Autodesk Inventor part; units mm, degrees
ref_plane "YZ Plane" through (0, 0, 0) normal (1, 0, 0) x (0, 1, 0)
ref_plane "XZ Plane" through (0, 0, 0) normal (0, 1, 0) x (-1, 0, 0)
ref_plane "XY Plane" through (0, 0, 0) normal (0, 0, 1) x (1, 0, 0)
sketch "Эскиз1" plane through (0, 0, 0) normal (0, 0, 1) x (1, 0, 0)
  circle A0 centre (0, 0) radius 3
  circle A1 centre (0, 0) radius 5
  dimension "d0" = 6
  dimension "d1" = 10
extrude "Выдавливание1" add sketch "Эскиз1" along normal blind 45
sketch "Эскиз2" plane through (0, 0, 0) normal (0, 0, -1) x (-1, 0, 0)
  circle A0 centre (0, 0) radius 13
  circle A1 centre (0, 0) radius 5
  circle A2 centre (0, 0) radius 3
  dimension "d4" = 26
extrude "Выдавливание2" add sketch "Эскиз2" along normal blind 3 contours A0 | A1
sketch "Эскиз3" plane through (0, 0, -3) normal (0, 0, -1) x (-1, 0, 0)
  circle A0 centre (0, 9) radius 1.5
  circle A1 centre (-9, 0) radius 1.5
  circle A2 centre (0, -9) radius 1.5
  circle A3 centre (9, 0) radius 1.5
  circle A4 centre (0, 0) radius 5
  dimension "d7" = 3
  dimension "d8" = 3
  dimension "d10" = 3
  dimension "d23" = 3
  dimension "d24" = 9
  dimension "d25" = 9
  dimension "d26" = 9
  dimension "d27" = 9
extrude "Выдавливание3" add sketch "Эскиз3" along normal blind 5 contours A0 | A1 | A2 | A3
fillet "Сопряжение1" radius 1 4 edges at (1.5, 9, -8) (10.5, 0, -8) (1.5, -9, -8) (-7.5, 0, -8)
sketch "Эскиз4" plane through (0, 0, 45) normal (0, 0, 1) x (1, 0, 0)
  circle A0 centre (0, 9) radius 1.5
  circle A1 centre (0, 0) radius 13
  circle A2 centre (0, 0) radius 5
  circle A3 centre (0, 0) radius 3
  point P0 (-0.5792, 4.9663)
  point P1 (0.5792, 4.9663)
extrude "Выдавливание4" add sketch "Эскиз4" along normal blind 3 contours A0 | A1 | A2
sketch "Эскиз6" plane through (0, 0, 48) normal (0, 0, 1) x (1, 0, 0)
  circle A0 centre (0, 0) radius 9.5
  circle A1 centre (0, 0) radius 13
  dimension "d19" = 19
extrude "Выдавливание6" add sketch "Эскиз6" along normal blind 5
sketch "Эскиз8" plane through (0, 0, 53) normal (0, 0, 1) x (1, 0, 0)
  circle A0 centre (-16.4751, 0) radius 1.5
  circle A1 centre (0, 9) radius 1.5
  arc A2 (1.4487, -9.3889) -> (-1.4487, -9.3889) centre (0, -9) ccw
  line L0 (0, 9) -> (0, -9)
  circle A3 centre (0, 0) radius 13
  circle A4 centre (0, 0) radius 9.5
  line L1 (-13, 2.5984) -> (-11.6906, 2.5984)
  line L2 (-13, -2.5984) -> (-12.3453, -2.5984)
  line L3 (-13, -2.5984) -> (-13, 2.5984)
  line L4 (-19.9502, -2.5984) -> (-13, -2.5984)
  line L5 (-19.9502, 2.5984) -> (-19.9502, -2.5984)
  line L6 (-19.9502, -2.5984) -> (-13, 2.5984) construction
  line L7 (-13, -2.5984) -> (-19.9502, 2.5984) construction
  line L8 (-13, 2.5984) -> (-19.9502, 2.5984)
  circle A5 centre (16.4751, 0) radius 1.5
  line L9 (13, 2.5984) -> (11.6906, 2.5984)
  line L10 (13, -2.5984) -> (12.3453, -2.5984)
  line L11 (13, -2.5984) -> (13, 2.5984)
  circle A6 centre (16.4751, 0) radius 1.5
  line L12 (19.9502, -2.5984) -> (13, -2.5984)
  line L13 (13, 2.5984) -> (19.9502, 2.5984)
  line L14 (19.9502, -2.5984) -> (13, 2.5984) construction
  line L15 (13, -2.5984) -> (19.9502, 2.5984) construction
  line L16 (19.9502, 2.5984) -> (19.9502, -2.5984)
  point P0 (12.7377, 2.5984)
  point P1 (12.7377, -2.5984)
  point P2 (-12.7377, -2.5984)
  point P3 (-12.7377, 2.5984)
  dimension "d30" = 3
extrude "Выдавливание7" add sketch "Эскиз8" against normal blind 3 contours L11 L10 A3 | L11 L13 L16 L12 | A3 L9 L11 | A3 L3 L1 | L2 L3 A3 | L3 L4 L5 L8
properties part number "вт1"
Verification items for the finished model (mm, model axes). A direction names the side the tool comes from. Round coordinates to 2 decimals unless told otherwise and drop trailing zeros. Order: outer loops, then holes, each group sorted by start corner. A loop starts at its lowest first (then second) coordinate and runs counter-clockwise, first axis right, second up. Notation, with made-up numbers: (88, 68.5) - (132, 68.5) arc R25 cw to (132, 97.5) - close; hole circle Ø4 at (-35, -4.5). An arc over 180 degrees is marked (long way). Use CSV: the item, a comma, the result in double quotes. Start each with the question number.
1) Mould release check, pull along Y, two halves, no side actions. Record for faces 5 (the flat face through (-2.24, 2.24, 48)), 6 (the flat face through (16, -2.598, 52)), 7 (the cylindrical face through (10.5, -0.07, -4.97)): +Y half, -Y half, draft (parallel to the pull), parting line (faces both ways), or undercut.
2) Section check A-A, the plane z = 47. Record the cut outline in (x, y).
3) Section check B-B, the plane z = 17. Record the cut outline in (x, y).
4) Thickness scan on L1, parallel to Z at x = 9.5, y = 6.25; L2, parallel to Z at x = -4, y = 6; L3, parallel to Y at x = 0, z = 50.6. Record the ranges inside material, lowest first.
5) Go/stop test with flat-tipped pins: P1, Ø6, axis at y = -9.5, z = 18, coming from the -X side; P2, Ø4, axis at x = 16, y = -1, coming from the -Z side; P3, Ø1.5, axis at x = -18, z = 52, coming from the +Y side; P4, Ø2.5, axis at x = 17.5, z = 52, coming from the -Y side. Record where each tip stops, or that it passes through.
6) Access from +Z, -Z, +X, -X, +Y, -Y to the whole of each face (thin tool, end or side, straight path). Record for faces 1 (the flat face through (-16, -2.598, 52)), 2 (the cylindrical face through (0.325, -7.536, -4.972)), 3 (the flat face through (-16, 2.598, 52)), 4 (the flat face through (-6, 0, 0)).
Answers:
1,face 5,"undercut"
1,face 6,"-Y half"
1,face 7,"parting line"
2,outline,"circle Ø26 at (0, 0); hole circle Ø6 at (0, 0)"
3,outline,"circle Ø10 at (0, 0); hole circle Ø6 at (0, 0)"
4,L1,"z = -3 to 0, 45 to 53"
4,L2,"z = -3 to 0, 45 to 48"
4,L3,"y = -13 to -9.5, 9.5 to 13"
5,P1,"passes through"
5,P2,"stops at z = 50"
5,P3,"stops at y = 2.6"
5,P4,"stops at y = -2.6"
6,face 1,"+Z, -Z, -X, -Y"
6,face 2,"-Z"
6,face 3,"+Z, -Z, -X, +Y"
6,face 4,"none"
